```python
from build123d import *

# Parameters (mm, degrees)
F1_DEPTH       = 25.4
F2_D           = 12.7
F2_CBORE_D     = 19.05
F2_CBORE_DEPTH = 6.35
F3_D           = 15.24
F4_D           = 12.7
F4_CSINK_D     = 25.4
F4_CSINK_ANGLE = 82
F5_D           = 10.16
F5_CBORE_D     = 20.32
F5_CBORE_DEPTH = 6.35


with BuildPart() as f1:
    # F0 (on Front) → F1 (new body)
    with BuildSketch(Plane.XZ):
        Polygon((0, 25.4), (0, 0), (127, 0), (127, 50.8), (0, 50.8), align=None)
    extrude(amount=F1_DEPTH)

    # F2 (through all)
    with Locations(Plane(origin=(0, 0, 0), x_dir=(1, 0, 0), z_dir=(0, 1, 0))):
        with Locations((107.95, -25.4)):
            CounterBoreHole(F2_D / 2, F2_CBORE_D / 2, F2_CBORE_DEPTH)

    # F3 (through all)
    with Locations(Plane(origin=(0, 0, 0), x_dir=(1, 0, 0), z_dir=(0, 1, 0))):
        with Locations((76.2, -25.4)):
            Hole(F3_D / 2)

    # F4 (through all)
    with Locations(Plane(origin=(0, 0, 0), x_dir=(1, 0, 0), z_dir=(0, 1, 0))):
        with Locations((44.45, -25.4)):
            CounterSinkHole(F4_D / 2, F4_CSINK_D / 2, counter_sink_angle=F4_CSINK_ANGLE)

    # F5 (through all)
    with Locations(Plane(origin=(0, 0, 0), x_dir=(1, 0, 0), z_dir=(0, 1, 0))):
        with Locations((19.05, -25.4)):
            CounterBoreHole(F5_D / 2, F5_CBORE_D / 2, F5_CBORE_DEPTH)


solid = f1.part
```
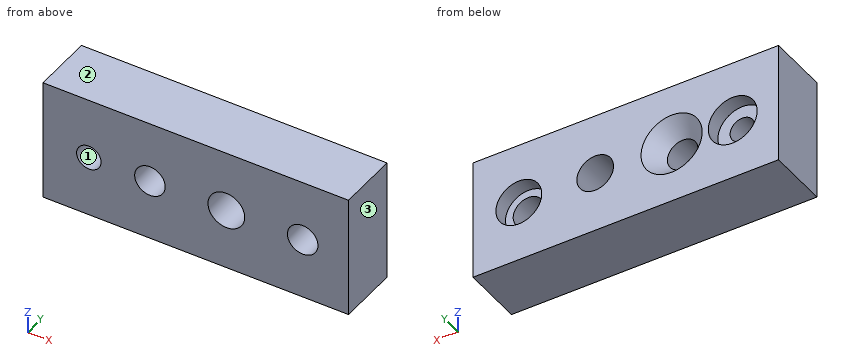
Geometry check sheet. Reference: the model listing, model coordinates, mm. Face numbers are marked on the shaded views. Coordinates: 2 decimals unless noted, no trailing zeros. Order: outer loops, then holes, each group sorted by start corner. A loop starts at its lowest first (then second) coordinate and runs counter-clockwise, first axis right, second up. Notation, with made-up numbers: M 85,41 L 122,41 A25 cw 122,53 Z; hole C 3,7 d4. An arc over 180 degrees is marked long. Answer as a JSON object with one key per item and string values.
Q1. Scan lines: line 1 (Z direction, x = 19.05, y = -11); line 2 (X direction, y = -14.75, z = 23.5); line 3 (Y direction, x = 99, z = 25). Record each from-to range of solid material in increasing order.
Results are:
{"line 1": "z = 0 to 20.32, 30.48 to 50.8", "line 2": "x = 0 to 14.34, 23.76 to 38.39, 50.51 to 68.82, 83.58 to 101.89, 114.01 to 127", "line 3": "y = -25.4 to -6.35"}
Q2. Cross-section at A-A on z = 25.4. Give the number of separate pieces and of enclosed holes in the cut face, and give its area (3 significant figures).
Results are:
{"separate pieces": "5", "enclosed holes": "0", "area": "1,780 mm²"}
Q3. Cross-section at D-D on x = 76.2. Record the cut outline in (y, z).
Results are:
{"outline": "M -25.4,0 L 0,0 L 0,17.78 L -25.4,17.78 Z; M -25.4,33.02 L 0,33.02 L 0,50.8 L -25.4,50.8 Z"}
Q4. Depth check by flat-ended pin: pin 1 Ø16.5 at (x, z) = (44.45, 25.4) entering from -Y; pin 2 Ø9 at (x, z) = (76.2, 25.4) entering from -Y; pin 3 Ø10 at (x, z) = (21, 28) entering from +Y. Enter the tip coordinate at first touch or a pass-through.
Results are:
{"pin 1": "stops at y = -25.4", "pin 2": "passes through", "pin 3": "stops at y = -6.35"}
Q5. Cross-section at C-C on x = 107.95. Record the cut outline in (y, z) (3 decimals), and give its area (3 significant figures).
Results are:
{"outline": "M -25.4,0 L 0,0 L 0,15.875 L -6.35,15.875 L -6.35,19.05 L -25.4,19.05 Z; M -25.4,31.75 L -6.35,31.75 L -6.35,34.925 L 0,34.925 L 0,50.8 L -25.4,50.8 Z", "area": "927 mm²"}
Q6. Cross-section at B-B on x = 19.05. Record the cut outline in (y, z), and give its area (3 significant figures).
Results are:
{"outline": "M -25.4,0 L 0,0 L 0,15.24 L -6.35,15.24 L -6.35,20.32 L -25.4,20.32 Z; M -25.4,30.48 L -6.35,30.48 L -6.35,35.56 L 0,35.56 L 0,50.8 L -25.4,50.8 Z", "area": "968 mm²"}
Q7. Release check for a two-part mould opening along Z. For the marked faces 1, 2 and 3 record: released by +Z, released by -Z, zero draft, split by the parting line, or undercut.
Results are:
{"face 1": "undercut", "face 2": "released by +Z", "face 3": "zero draft"}
